Answer from the drawing. Dimensions are ordinates in mm from the lowest x, y and z of the part. A direction names the side the tool comes from. Coordinates: 2 decimals unless noted, no trailing zeros. Loops run counter-clockwise (first coordinate to the right, second up) from the corner with the lowest first, then second, coordinate; pieces in that order, holes last. Notation, with made-up numbers: (20, 21) -> (49, 21) arc R13 cw to (49, 32) -> close; hole circle Ø4 at (3, -17). An arc over 180 degrees is marked (long way). Answer as CSV lines item,"result".
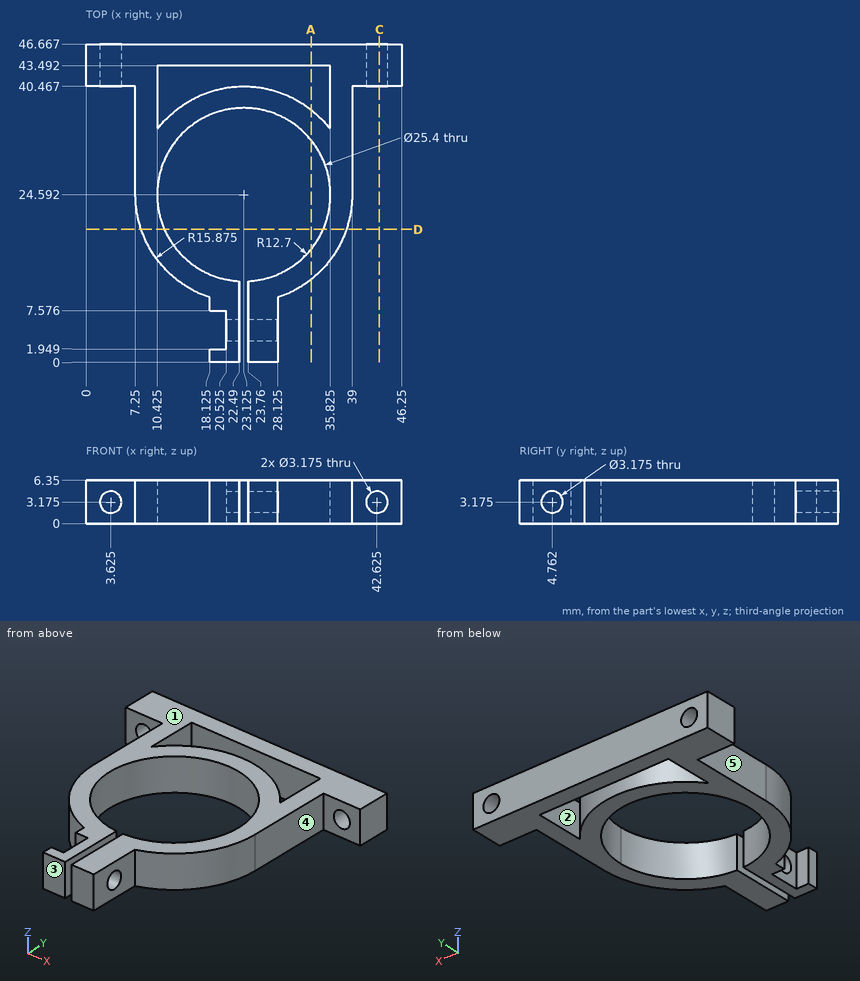
(1) Which of the six approach directions +Z, -Z, +X, -X, +Y, -Y give full straight-line access (tool end or side, diameter ignored) to the marked faces 1, 2, 3, 4 and 5?
Computed values:
face 1,"+Z, +X, -X, +Y, -Y"
face 2,"+Z, -Z"
face 3,"+Z, -Z, +X, -X, -Y"
face 4,"+Z, -Z, +X, -Y"
face 5,"+Z, -Z, -X, -Y"
(2) Consider line 1 along Y through (x, z) = (28.5, 3) (1 decimal); line 2 along X through (y, z) = (44.5, 3); line 3 along Y through (x, z) = (13, 1) (1 decimal). Determine where each line is inside the solid, lowest interval first.
Computed values:
line 1,"9.7 to 13.1, 36.1 to 39.5, 43.5 to 46.7"
line 2,"0 to 2.05, 5.2 to 41.05, 44.2 to 46.25"
line 3,"12.4 to 16.9, 32.3 to 36.8, 43.5 to 46.7"
(3) Flat-ended cylindrical pins translate along their axes: pin 1 Ø1.9 at (y, z) = (4.5, 2) entering from +X (1 decimal); pin 2 Ø2 at (x, y) = (12.5, 18.5) entering from -Z; pin 3 Ø3.5 at (x, z) = (42.625, 3.175) entering from -Y; pin 4 Ø3 at (y, z) = (5.5, 4.5) entering from -X (1 decimal). Find the tip coordinate at first contact, or state that the pin passes through.
Computed values:
pin 1,"x = 28.1"
pin 2,"z = 0"
pin 3,"y = 40.47"
pin 4,"x = 20.5"
(4) A cutting plane is placed at A-A, the plane x = 33. Write down the section's boundary in (y, z).
Computed values:
outline,"(12.16, 0) -> (16.61, 0) -> (16.61, 6.35) -> (12.16, 6.35) -> close; (32.58, 0) -> (37.02, 0) -> (37.02, 6.35) -> (32.58, 6.35) -> close; (43.49, 0) -> (46.67, 0) -> (46.67, 6.35) -> (43.49, 6.35) -> close"
(5) A cutting plane is placed at D-D, the plane y = 19.5. Write down the section's boundary in (x, z), and give its area (3 significant figures).
Computed values:
outline,"(8.09, 0) -> (11.49, 0) -> (11.49, 6.35) -> (8.09, 6.35) -> close; (34.76, 0) -> (38.16, 0) -> (38.16, 6.35) -> (34.76, 6.35) -> close"
area,"43.2 mm2"
(6) A cutting plane is placed at C-C, the plane x = 43. Write down the section's boundary in (y, z).
Computed values:
outline,"(40.47, 0) -> (46.67, 0) -> (46.67, 1.63) -> (40.47, 1.63) -> close; (40.47, 4.72) -> (46.67, 4.72) -> (46.67, 6.35) -> (40.47, 6.35) -> close"
